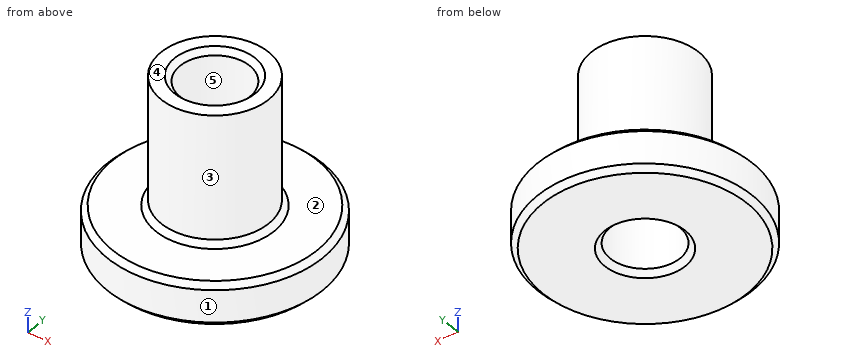
```python
from build123d import *

# Parameters (mm, degrees)
F0_R     = 15.875
F1_DEPTH = 25.4
F2_D     = 10.3
F3_SIZE  = 0.79375
F4_SIZE  = 0.79375
F5_R     = 15.875
F5_R_2   = 7.9375
F6_DEPTH = 19.05
F7_SIZE  = 0.79375


with BuildPart() as f1:
    # F0 (on Top) → F1 (new body)
    with BuildSketch(Plane.XY):
        Circle(F0_R)
    extrude(amount=F1_DEPTH)

    # F2 (through all)
    with Locations(Plane(origin=(0, 0, 0), x_dir=(1, 0, 0), z_dir=(0, 0, -1))):
        with Locations((0, 0)):
            Hole(F2_D / 2)

    # F3
    f3_edges = [f1.edges().sort_by_distance(p)[0] for p in [
        (-15.875, 0, 0),
    ]]
    chamfer(f3_edges, length=F3_SIZE)

    # F4
    f4_edges = [f1.edges().sort_by_distance(p)[0] for p in [
        (-15.875, 0, 25.4),
        (-5.15, 0, 25.4),
        (-5.15, 0, 0),
    ]]
    chamfer(f4_edges, length=F4_SIZE)

    # F5 (on face) → F6 (cut)
    with BuildSketch(Plane.XY.offset(25.4)):
        Circle(F5_R)
        Circle(F5_R_2, mode=Mode.SUBTRACT)
    extrude(amount=-F6_DEPTH, mode=Mode.SUBTRACT)

    # F7
    f7_edges = [f1.edges().sort_by_distance(p)[0] for p in [
        (-15.875, 0, 6.35),
        (-7.9375, 0, 6.35),
    ]]
    chamfer(f7_edges, length=F7_SIZE)


solid = f1.part
```
Input: part model. Units: mm. Frame: model coordinates. Face numbers are marked on the shaded views. A direction names the side the tool comes from. Give positions to 0.01 mm unless a question says otherwise; leave off trailing zeros.
1. Draft query along X for the marked faces 3, 4 and 5. Return one class per face: released by +X, released by -X, zero draft, split by the parting line, or undercut.
Computed:
face 3: split by the parting line
face 4: zero draft
face 5: undercut
2. Set-up query: the marked faces 1 and 2. Return all of +Z, -Z, +X, -X, +Y, -Y with unobstructed straight access to the full face (end or side cutting, diameter ignored); none if empty.
Computed:
face 1: +Z, -Z
face 2: +Z
3. Line query: probe 1 along Y at (x, z) = (0, 10.25); probe 2 along Z at (x, y) = (-6.5, -8); probe 3 along Y at (x, z) = (-1.5, 21.75). Output: solid intervals per line, ascending.
Computed:
probe 1: y = -7.94 to -5.15, 5.15 to 7.94
probe 2: z = 0 to 6.35
probe 3: y = -7.79 to -4.93, 4.93 to 7.79
4. Pin query (flat end, axial travel): pin 1 Ø8 at (x, z) = (2.5, 18) entering from -Y; pin 2 Ø3 at (x, z) = (10, 19) entering from +Y; pin 3 Ø2 at (x, z) = (8, 6.5) entering from +Y; pin 4 Ø2 at (y, z) = (-2.5, 6.5) entering from +X. Return the tip coordinate at first contact, or that it passes through.
Computed:
pin 1: stops at y = -7.94
pin 2: passes through
pin 3: stops at y = 13.91
pin 4: stops at x = 15.73
